Autodesk Inventor part; units mm, degrees
ref_plane "YZ Plane" through (0, 0, 0) normal (1, 0, 0) x (0, 1, 0)
ref_plane "XZ Plane" through (0, 0, 0) normal (0, 1, 0) x (-1, 0, 0)
ref_plane "XY Plane" through (0, 0, 0) normal (0, 0, 1) x (1, 0, 0)
sketch "Эскиз1" plane through (0, 0, 0) normal (0, 1, 0) x (-1, 0, 0)
  line L0 (0, 0) -> (120, 0)
  line L1 (120, 0) -> (120, -20)
  line L2 (120, -20) -> (0, -20)
  line L3 (0, -20) -> (0, 0)
  dimension "d0" = 20
  dimension "d1" = 120
sketch "Эскиз2" plane through (0, 0, 0) normal (0, 1, 0) x (-1, 0, 0)
  line L0 (0, -20) -> (15, -20)
  line L1 (15, -20) -> (15, -16)
  line L2 (15, -16) -> (0, -16)
  line L3 (0, -16) -> (0, -20)
  line L4 (120, -20) -> (105, -20)
  line L5 (105, -20) -> (105, -16)
  line L6 (105, -16) -> (120, -16)
  line L7 (120, -16) -> (120, -20)
  point P0 (0, 0)
  dimension "d2" = 15
  dimension "d3" = 4
  dimension "d39" = 15
  dimension "d40" = 90
  dimension "d41" = 16
  dimension "d42" = 4
  dimension "d43" = 15
  dimension "d44" = 16
extrude "Выдавливание1" add sketch "Эскиз1" along normal blind 4
sketch "Эскиз3" plane through (0, 4, 0) normal (0, 1, 0) x (1, 0, 0)
  circle A0 centre (-111.5, 10) radius 3.05
  line L0 (-120, 0) -> (0, 0)
  line L1 (-120, 20) -> (-120, 0)
  circle A1 centre (-8.5, 10) radius 3.05
  line L2 (0, 0) -> (0, 20)
  point P0 (0, 16)
  dimension "d9" = 6.1
  dimension "d14" = 10
  dimension "d27" = 8.5
  dimension "d28" = 6.1
  dimension "d29" = 8.5
  dimension "d30" = 10
sketch "Эскиз4" plane through (0, 4, 0) normal (0, 1, 0) x (1, 0, 0)
  circle A0 centre (-8.5, 10) radius 5.1
  line L0 (-120, 0) -> (0, 0)
  line L1 (0, 0) -> (0, 20)
  circle A1 centre (-111.5, 10) radius 5.1
  line L2 (-120, 20) -> (-120, 0)
  point P0 (0, 16)
  dimension "d11" = 10.2
  dimension "d12" = 10
  dimension "d33" = 8.5
  dimension "d34" = 10.2
  dimension "d35" = 8.5
  dimension "d36" = 10
extrude "Выдавливание6" cut sketch "Эскиз3" against normal blind 10
extrude "Выдавливание7" cut sketch "Эскиз4" against normal blind 2.4
extrude "Выдавливание8" add sketch "Эскиз2" along normal blind 21
sketch "Эскиз6" plane through (-120, 4, -16) normal (0, 0, 1) x (1, 0, 0)
  circle A0 centre (7.5, 7.5) radius 3.05
  circle A1 centre (112.5, 7.5) radius 3.05
  line L0 (0, 0) -> (120, 0)
  line L1 (0, 0) -> (0, 17)
  line L2 (105, 0) -> (105, 17)
  line L3 (120, 0) -> (120, 17)
  point P0 (120, -4)
  point P1 (0, 15)
  point P2 (105, 15)
  point P3 (120, 15)
  dimension "d48" = 6.1
  dimension "d49" = 6.1
  dimension "d50" = 7.5
  dimension "d51" = 7.5
  dimension "d53" = 7.5
  dimension "d66" = 7.5
sketch "Эскиз7" plane through (-17, 4, -20) normal (0, 0, 1) x (1, 0, 0)
  circle A0 centre (9.5, 7.5) radius 5.1
  circle A1 centre (-95.5, 7.5) radius 5.1
  line L0 (-103, 0) -> (17, 0)
  line L1 (-88, 0) -> (-88, 17)
  line L2 (17, 0) -> (17, 17)
  line L3 (-103, -4) -> (-103, 17)
  point P0 (17, -4)
  point P1 (-88, 15)
  point P2 (17, 15)
  point P3 (-103, 15)
  dimension "d54" = 10.2
  dimension "d55" = 10.2
  dimension "d56" = 7.5
  dimension "d58" = 7.5
  dimension "d59" = 7.5
  dimension "d67" = 7.5
extrude "Выдавливание9" cut sketch "Эскиз6" against normal blind 21
fillet "Сопряжение4" radius 1 1 edges at (-116.6, 1.6, -10)
sketch "Эскиз8" plane through (-120, 0, 0) normal (0, 0, 1) x (1, 0, 0)
  point P0 (120, 0)
sketch "Эскиз9" plane through (0, 0, 0) normal (0, -1, 0) x (1, 0, 0)
  line L0 (-120, 0) -> (0, 0)
  line L1 (0, 0) -> (6, 0)
  line L2 (6, 0) -> (6, -20)
  line L3 (6, -20) -> (0, -20)
  line L4 (0, -20) -> (0, 0)
  line L5 (-120, 0) -> (-126, 0)
  line L6 (-126, 0) -> (-126, -20)
  line L7 (-126, -20) -> (-120, -20)
  line L8 (-120, -20) -> (-120, 0)
  dimension "d68" = 6
  dimension "d69" = 6
  dimension "d70" = 20
  dimension "d71" = 120
  dimension "d72" = 20
extrude "Выдавливание11" add sketch "Эскиз9" against normal blind 124
sketch "Эскиз10" plane through (0, 124, 0) normal (0, 1, 0) x (1, 0, 0)
  line L0 (6, 0) -> (6, 20)
  line L1 (-126, 20) -> (6, 20)
  line L2 (6, 0) -> (-126, 0)
  line L3 (-126, 0) -> (-126, 20)
  line L4 (-126, 20) -> (6, 20)
  line L5 (6, 20) -> (6, 0)
  point P0 (0, 0)
extrude "Выдавливание12" add sketch "Эскиз10" along normal blind 6
sketch "Эскиз11" plane through (-126, 0, -20) normal (-1, 0, 0) x (0, 0, 1)
  line L0 (0, 0) -> (20, 0)
  line L1 (0, 130) -> (20, 130)
  line L2 (7.75, 0) -> (12.25, 0)
  line L3 (12.25, 0) -> (12.25, 130)
  line L4 (12.25, 130) -> (7.75, 130)
  line L5 (7.75, 130) -> (7.75, 0)
  line L6 (20, 0) -> (20, 130)
  dimension "d77" = 4.5
  dimension "d78" = 7.75
sketch "Эскиз12" plane through (6, 0, 0) normal (1, 0, 0) x (0, 0, -1)
  line L0 (20, 0) -> (0, 0)
  line L1 (20, 130) -> (0, 130)
  line L2 (7.75, 0) -> (12.25, 0)
  line L3 (12.25, 0) -> (12.25, 130)
  line L4 (12.25, 130) -> (7.75, 130)
  line L5 (7.75, 130) -> (7.75, 0)
  line L6 (20, 0) -> (20, 130)
  dimension "d79" = 4.5
  dimension "d80" = 7.75
extrude "Выдавливание13" cut sketch "Эскиз11" against normal blind 4.5 contours L5 L1 L3 L0
extrude "Выдавливание14" cut sketch "Эскиз12" against normal blind 4.5 contours L0 L5 L1 L3
sketch "Эскиз13" plane through (0, 130, 0) normal (0, 1, 0) x (1, 0, 0)
  line L0 (-121.5, 12.25) -> (-121.5, 7.75)
  line L1 (1.5, 7.75) -> (1.5, 12.25)
  line L2 (-121.5, 7.75) -> (1.5, 7.75)
  line L3 (1.5, 7.75) -> (1.5, 12.25)
  line L4 (1.5, 12.25) -> (-121.5, 12.25)
  line L5 (-121.5, 12.25) -> (-121.5, 7.75)
  point P0 (0, 0)
extrude "Выдавливание15" cut sketch "Эскиз13" against normal blind 4.5
sketch "Эскиз15" plane through (0, 124, 0) normal (0, -1, 0) x (1, 0, 0)
  line L0 (0, -20) -> (-120, -20)
  line L1 (-120, -20) -> (-105, -20)
  line L2 (-105, -20) -> (-105, -16)
  line L3 (-105, -16) -> (-120, -16)
  line L4 (-120, -16) -> (-120, -20)
  line L5 (0, -20) -> (-15, -20)
  line L6 (-15, -20) -> (-15, -16)
  line L7 (-15, -16) -> (0, -16)
  line L8 (0, -16) -> (0, -20)
  point P0 (0, 0)
  dimension "d87" = 15
  dimension "d88" = 4
  dimension "d89" = 15
  dimension "d90" = 4
extrude "Выдавливание16" add sketch "Эскиз15" along normal blind 17
sketch "Эскиз16" plane through (-120, 124, -16) normal (0, 0, 1) x (1, 0, 0)
  circle A0 centre (7.5, -7.5) radius 3.05
  circle A1 centre (112.5, -7.5) radius 3.05
  line L0 (0, -17) -> (0, 0)
  line L1 (0, 0) -> (15, 0)
  line L2 (105, 0) -> (120, 0)
  line L3 (120, 0) -> (120, -17)
  point P0 (120, -124)
  dimension "d93" = 6.1
  dimension "d94" = 6.1
  dimension "d95" = 7.5
  dimension "d96" = 7.5
  dimension "d97" = 7.5
  dimension "d98" = 7.5
extrude "Выдавливание17" cut sketch "Эскиз16" against normal blind 17
sketch "Эскиз17" plane through (6, 0, -20) normal (0, 0, -1) x (-1, 0, 0)
  circle A0 centre (13.5, 116.5) radius 5.1
  circle A1 centre (118.5, 116.5) radius 3.05
  circle A2 centre (118.5, 116.5) radius 5.1
  line L0 (21, 124) -> (21, 107)
  line L1 (21, 124) -> (111, 124)
  line L2 (111, 124) -> (111, 107)
  point P0 (6, 0)
  dimension "d101" = 10.2
  dimension "d102" = 10.2
  dimension "d103" = 7.5
  dimension "d104" = 7.5
  dimension "d105" = 7.5
  dimension "d106" = 7.5
fillet "Сопряжение9" radius 2 8 edges at (-105, 107, -18) (-105, 21, -18) (-15, 107, -18) (-15, 21, -18) (6, 130, -3.875) (6, 130, -16.125) (-126, 130, -3.875) (-126, 130, -16.125)
properties part number "КрепежКулера"
For this review, take the finished solid that the model builds, in its own axes (mm). A direction names the side the tool comes from. Coordinates: 2 decimals unless noted, no trailing zeros. Loops run counter-clockwise (first coordinate to the right, second up) from the corner with the lowest first, then second, coordinate; pieces in that order, holes last. Notation, with made-up numbers: (68.25, 19.5) - (100.25, 19.5) arc R17 ccw to (100.25, 30.5) - close; hole circle Ø5 at (1, -18.75). An arc over 180 degrees is marked (long way). Return JSON: item names as keys, results as strings.
Item 1: Take a section at A-A (x = -44.5). Give the boundary of the cut face in (y, z), then the cut area to 3 significant figures.
Determined:
{"outline": "(0, -20) - (4, -20) - (4, 0) - (0, 0) - close; (124, -20) - (130, -20) - (130, -12.25) - (125.5, -12.25) - (125.5, -7.75) - (130, -7.75) - (130, 0) - (124, 0) - close", "area": "180 mm2"}
Item 2: For faces 1 (the flat face through (-126, 63, -16)), 2 (the flat face through (1.5, 64, -10)), 3 (the flat face through (-15, 11, -18)), 4 (the flat face through (0, 63, -10)), 5 (the flat face through (-6, 1.6, -8)), list the 3-axis set-ups (+Z, -Z, +X, -X, +Y, -Y) from which the entire face can be reached by the end or side of a thin tool; tool diameter is ignored.
Determined:
{"face 1": "+Z, -Z, -X, +Y, -Y", "face 2": "+X, +Y, -Y", "face 3": "+Z, -Z", "face 4": "+Z", "face 5": "none"}
Item 3: Take a section at C-C (y = 58). Give the boundary of the cut face in (x, z), then the cut area to 4 significant figures.
Determined:
{"outline": "(-126, -20) - (-120, -20) - (-120, 0) - (-126, 0) - (-126, -7.75) - (-121.5, -7.75) - (-121.5, -12.25) - (-126, -12.25) - close; (0, -20) - (6, -20) - (6, -12.25) - (1.5, -12.25) - (1.5, -7.75) - (6, -7.75) - (6, 0) - (0, 0) - close", "area": "199.5 mm2"}
Item 4: Mouldability with a two-part tool opening along X and no side actions: class faces 6 (the flat face through (-61, 130, -16)), 7 (the flat face through (-126, 63, -4)), 8 (the flat face through (-105, 117, -18)) as pulls with the +X half, pulls with the -X half, needs draft (parallel to the pull), parting line crosses it, or undercut.
Determined:
{"face 6": "needs draft", "face 7": "pulls with the -X half", "face 8": "undercut"}
Item 5: Take a section at D-D (y = 116.5). Give the boundary of the cut face in (x, z).
Determined:
{"outline": "(-126, -20) - (-115.55, -20) - (-115.55, -16) - (-120, -16) - (-120, 0) - (-126, 0) - (-126, -7.75) - (-121.5, -7.75) - (-121.5, -12.25) - (-126, -12.25) - close; (-109.45, -20) - (-105, -20) - (-105, -16) - (-109.45, -16) - close; (-15, -20) - (-10.55, -20) - (-10.55, -16) - (-15, -16) - close; (-4.45, -20) - (6, -20) - (6, -12.25) - (1.5, -12.25) - (1.5, -7.75) - (6, -7.75) - (6, 0) - (0, 0) - (0, -16) - (-4.45, -16) - close"}
Item 6: For line 1 (X direction, y = 3.65, z = -10); line 2 (Y direction, x = -112.5, z = -18.8); line 3 (X direction, y = 0.7, z = -10), list the stretches that pass through material, from the lowest coordinate up.
Determined:
{"line 1": "x = -121.5 to -116.6, -106.4 to -13.6, -3.4 to 1.5", "line 2": "y = 0 to 8.45, 14.55 to 21, 107 to 113.45, 119.55 to 130", "line 3": "x = -121.5 to -114.55, -108.45 to -11.55, -5.45 to 1.5"}
Item 7: Insertion check: pin 1 (3.5 mm diameter, centred on x = -8.5, z = -10, fed in from +Y); pin 2 (5.5 mm diameter, centred on x = -112.5, y = 116.5, fed in from +Z); pin 3 (3.5 mm diameter, centred on y = 92, z = -10, fed in from -X). Each pin has a flat end and moves straight along its axis. Give the tip position at first contact, or say it passes through.
Determined:
{"pin 1": "stops at y = 125.5", "pin 2": "passes through", "pin 3": "stops at x = -121.5"}
Item 8: Take a section at B-B (z = -10). Give the boundary of the cut face in (x, y), then the cut area to 3 significant figures.
Determined:
{"outline": "(-121.5, 0) - (-114.55, 0) - (-114.55, 1.6) - (-115.6, 1.6) arc R1 cw to (-116.6, 2.6) - (-116.6, 4) - (-120, 4) - (-120, 124) - (0, 124) - (0, 4) - (-3.4, 4) - (-3.4, 1.6) - (-5.45, 1.6) - (-5.45, 0) - (1.5, 0) - (1.5, 125.5) - (-121.5, 125.5) - close; (-108.45, 0) - (-11.55, 0) - (-11.55, 1.6) - (-13.6, 1.6) - (-13.6, 4) - (-106.4, 4) - (-106.4, 2.6) arc R1 cw to (-107.4, 1.6) - (-108.45, 1.6) - close", "area": "968 mm2"}
